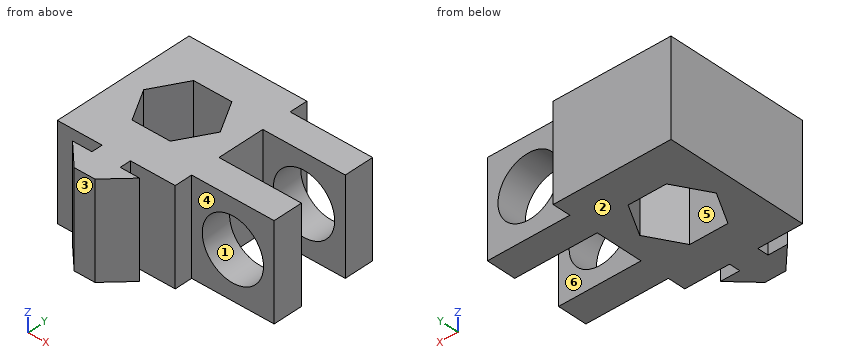
```python
from build123d import *

# Parameters (mm, degrees)
BOSS_EXTRUDE1_DEPTH = 10.16
SKETCH2_R           = 6.604
CUT_EXTRUDE1_DEPTH  = 38.916561489


with BuildPart() as part:
    # Sketch1 → Boss-Extrude1 (new body, symmetric)
    with BuildSketch(Plane.XY):
        Polygon((2.24536, 0), (-2.24536, 0), (-7.239, 4.99364), (-3.048, 4.99364), (-3.048, 7.366), (-12.7, 7.366), (-12.7, 37.916561489), (12.7, 37.916561489), (12.7, 34.036), (30.48, 34.036), (30.48, 27.686), (12.7, 27.686), (12.7, 17.526), (30.48, 17.526), (30.48, 11.176), (12.7, 11.176), (12.7, 7.366), (3.048, 7.366), (3.048, 4.99364), (7.239, 4.99364), align=None)
        Polygon((-4.124445986, 29.74975), (-8.248891971, 22.606), (-4.124445986, 15.46225), (4.124445986, 15.46225), (8.248891971, 22.606), (4.124445986, 29.74975), align=None, mode=Mode.SUBTRACT)
    extrude(amount=BOSS_EXTRUDE1_DEPTH, both=True)

    # Sketch2 → Cut-Extrude1 (cut, through all)
    with BuildSketch(Plane(origin=(0, 37.916561489, 0), x_dir=(1, 0, 0), z_dir=(0, 1, 0))):
        with Locations((21.59, 0)):
            Circle(SKETCH2_R)
    extrude(amount=-CUT_EXTRUDE1_DEPTH, mode=Mode.SUBTRACT)


solid = part.part
```
Design review of the part built by this model. Coordinates are the model's own, in mm. Face numbers are marked on the shaded views. A direction names the side the tool comes from. Give positions to 0.01 mm unless a question says otherwise; leave off trailing zeros. Order: outer loops, then holes, each group sorted by start corner. A loop starts at its lowest first (then second) coordinate and runs counter-clockwise, first axis right, second up. Notation, with made-up numbers: (8, 67) -> (52, 67) arc R29 cw to (52, 96) -> close; hole circle Ø5 at (8, -5). An arc over 180 degrees is marked (long way). Write each question's results on one line, items separated by ' | '. Start each with the question number.
Q1. For pin 1 (12 mm diameter, centred on x = 14, z = 7.5, fed in from -Y); pin 2 (5 mm diameter, centred on y = 24.5, z = 3, fed in from +X); pin 3 (7.5 mm diameter, centred on x = 8.5, z = 2.5, fed in from -Y), all flat-tipped, find the tip position at first contact; note any pin that passes through.
Q2. Add section A-A on x = 21.59. Give the boundary of the cut face in (y, z), and give its area (3 significant figures).
Q3. Add section C-C on x = -1. Give the boundary of the cut face in (y, z).
Q4. Add section B-B on z = 0. State how many separate pieces and enclosed holes the cut face has, and give its area (3 significant figures).
Q5. Mouldability with a two-part tool opening along Z and no side actions: class the marked faces 1, 2 and 3 as +Z half, -Z half, draft (parallel to the pull), parting line (faces both ways), or undercut.
Q6. Wall thickness on L1, parallel to Y at x = 3.5, z = -7.25; L2, parallel to Y at x = 29, z = -6.5; L3, parallel to Y at x = -5, z = -7.5: over which ranges is each line inside the solid? List them lowest first. Write a range as from..to.
Q7. Machinability: for the marked faces 4, 5 and 6, which of the approach directions +Z, -Z, +X, -X, +Y, -Y give a long, thin tool a straight path to every point of the face, cutting with its end or side? Answer none if there is none.
Q8. Add section D-D on y = 18.5. Give the boundary of the cut face in (x, z).
Found:
1) pin 1: stops at y = 7.37 | pin 2: stops at x = 12.7 | pin 3: stops at y = 2.5
2) outline: (11.18, -10.16) -> (17.53, -10.16) -> (17.53, -6.6) -> (11.18, -6.6) -> close; (11.18, 6.6) -> (17.53, 6.6) -> (17.53, 10.16) -> (11.18, 10.16) -> close; (27.69, -10.16) -> (34.04, -10.16) -> (34.04, -6.6) -> (27.69, -6.6) -> close; (27.69, 6.6) -> (34.04, 6.6) -> (34.04, 10.16) -> (27.69, 10.16) -> close | area: 90.3 mm2
3) outline: (0, -10.16) -> (15.46, -10.16) -> (15.46, 10.16) -> (0, 10.16) -> close; (29.75, -10.16) -> (37.92, -10.16) -> (37.92, 10.16) -> (29.75, 10.16) -> close
4) separate pieces: 3 | enclosed holes: 1 | area: 719 mm2
5) face 1: undercut | face 2: -Z half | face 3: draft
6) L1: y = 1.25..4.99, 7.37..15.46, 29.75..37.92 | L2: y = 11.18..17.53, 27.69..34.04 | L3: y = 2.75..4.99, 7.37..16.98, 28.23..37.92
7) face 4: +Z, -Z, +X, -Y | face 5: +Z, -Z | face 6: +Z, -Z, +X
8) outline: (-12.7, -10.16) -> (-5.88, -10.16) -> (-5.88, 10.16) -> (-12.7, 10.16) -> close; (5.88, -10.16) -> (12.7, -10.16) -> (12.7, 10.16) -> (5.88, 10.16) -> close
